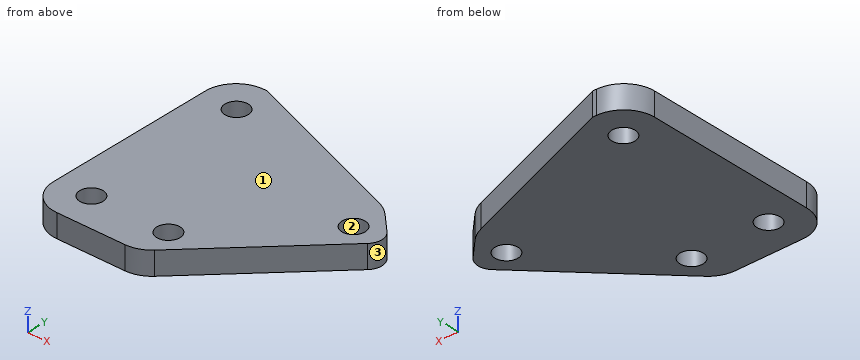
```python
from build123d import *

# Parameters (mm, degrees)
SKETCH1_R           = 1.5
BOSS_EXTRUDE1_DEPTH = 3
FILLET1_R           = 2
FILLET3_R           = 5
FILLET5_R           = 4
FILLET6_R           = 4
FILLET7_R           = 4


with BuildPart() as part:
    # Sketch1 → Boss-Extrude1 (new body)
    with BuildSketch(Plane.XY):
        Polygon((0, 0), (14.5, 0), (19, 4.5), (31.727922061, 17.227922061), (27.227922061, 21.727922061), (4.5, 30.213203436), (0, 30.213203436), align=None)
        with Locations((4.5, 25.713203436)):
            Circle(SKETCH1_R, mode=Mode.SUBTRACT)
        with Locations((4.5, 4.5)):
            Circle(SKETCH1_R, mode=Mode.SUBTRACT)
        with Locations((14.5, 4.5)):
            Circle(SKETCH1_R, mode=Mode.SUBTRACT)
        with Locations((27.227922061, 17.227922061)):
            Circle(SKETCH1_R, mode=Mode.SUBTRACT)
    extrude(amount=BOSS_EXTRUDE1_DEPTH)

    # Fillet1
    fillet1_edges = [part.edges().sort_by_distance(p)[0] for p in [
        (31.727922061, 17.227922061, 1.5),
    ]]
    fillet(fillet1_edges, radius=FILLET1_R)

    # Fillet3
    fillet3_edges = [part.edges().sort_by_distance(p)[0] for p in [
        (27.227922061, 21.727922061, 1.5),
    ]]
    fillet(fillet3_edges, radius=FILLET3_R)

    # Fillet5
    fillet5_edges = [part.edges().sort_by_distance(p)[0] for p in [
        (0, 30.213203436, 1.5),
    ]]
    fillet(fillet5_edges, radius=FILLET5_R)

    # Fillet6
    fillet6_edges = [part.edges().sort_by_distance(p)[0] for p in [
        (0, 0, 1.5),
    ]]
    fillet(fillet6_edges, radius=FILLET6_R)

    # Fillet7
    fillet7_edges = [part.edges().sort_by_distance(p)[0] for p in [
        (14.5, 0, 1.5),
    ]]
    fillet(fillet7_edges, radius=FILLET7_R)


solid = part.part
```
Check sheet for the modelled part. Datum: model origin and axes. Units: mm. Face numbers are marked on the shaded views. Coordinates: 2 decimals unless noted, no trailing zeros. Order: outer loops, then holes, each group sorted by start corner. A loop starts at its lowest first (then second) coordinate and runs counter-clockwise, first axis right, second up. Notation, with made-up numbers: M -10.75,57 L 22.25,57 A32 cw 22.25,89 Z; hole C -14.75,17 d9. An arc over 180 degrees is marked long. Write each question's results on one line, items separated by ' | '. Start each with the question number.
1. Cross-section at C-C on x = 14.5. Record the cut outline in (y, z), and give its area (3 significant figures).
2. Go/stop test with a flat-tipped pin: P1, Ø1, axis at y = 3.5, z = 2.5, coming from the +X side. Record where the tip stops, or that it passes through.
3. Cross-section at B-B on z = 1.95. Record the cut outline in (x, y).
4. Mould release check, pull along X, two halves, no side actions. Record for the marked faces 1, 2 and 3: +X half, -X half, draft (parallel to the pull), parting line (faces both ways), or undercut.
5. Cross-section at A-A on y = 4.5. Record the cut outline in (x, z).
6. Cross-section at D-D on y = 14.5. Record the cut outline in (x, z).
7. Material ranges on probe 1 along Y at (x, z) = (4.5, 1.45); probe 2 along Y at (x, z) = (5.5, 1.25); probe 3 along X at (y, z) = (13.5, 0.6), recorded low to high.
Checks:
1) outline: M 0.36,0 L 3,0 L 3,3 L 0.36,3 Z; M 6,0 L 26.48,0 L 26.48,3 L 6,3 Z | area: 69.4 mm²
2) P1: stops at x = 18.5
3) outline: M 0,4 A4 ccw 4,0 L 12.84,0 A4 ccw 15.67,1.17 L 30.31,15.81 A2 ccw 30.31,18.64 L 28,20.96 A5 ccw 26.21,22.11 L 4.5,30.21 L 4,30.21 A4 ccw 0,26.21 Z; hole C 4.5,4.5 d3; hole C 4.5,25.71 d3; hole C 14.5,4.5 d3; hole C 27.23,17.23 d3
4) face 1: draft | face 2: undercut | face 3: +X half
5) outline: M 0,0 L 3,0 L 3,3 L 0,3 Z; M 6,0 L 13,0 L 13,3 L 6,3 Z; M 16,0 L 19,0 L 19,3 L 16,3 Z
6) outline: M 0,0 L 29,0 L 29,3 L 0,3 Z
7) probe 1: y = 0 to 3, 6 to 24.21, 27.21 to 30.21 | probe 2: y = 0 to 3.38, 5.62 to 24.6, 26.83 to 29.84 | probe 3: x = 0 to 28
